Verification items for this drawing (mm, ordinates from the low corner). A direction names the side the tool comes from. Coordinates: 2 decimals unless noted, no trailing zeros. Loops run counter-clockwise (first coordinate to the right, second up) from the corner with the lowest first, then second, coordinate; pieces in that order, holes last. Notation, with made-up numbers: M 9,-23 L 66,-23 A17 cw 66,10 Z; hole C 76.5,51.25 d2. An arc over 180 degrees is marked long. Return JSON: item names as keys, results as strings.
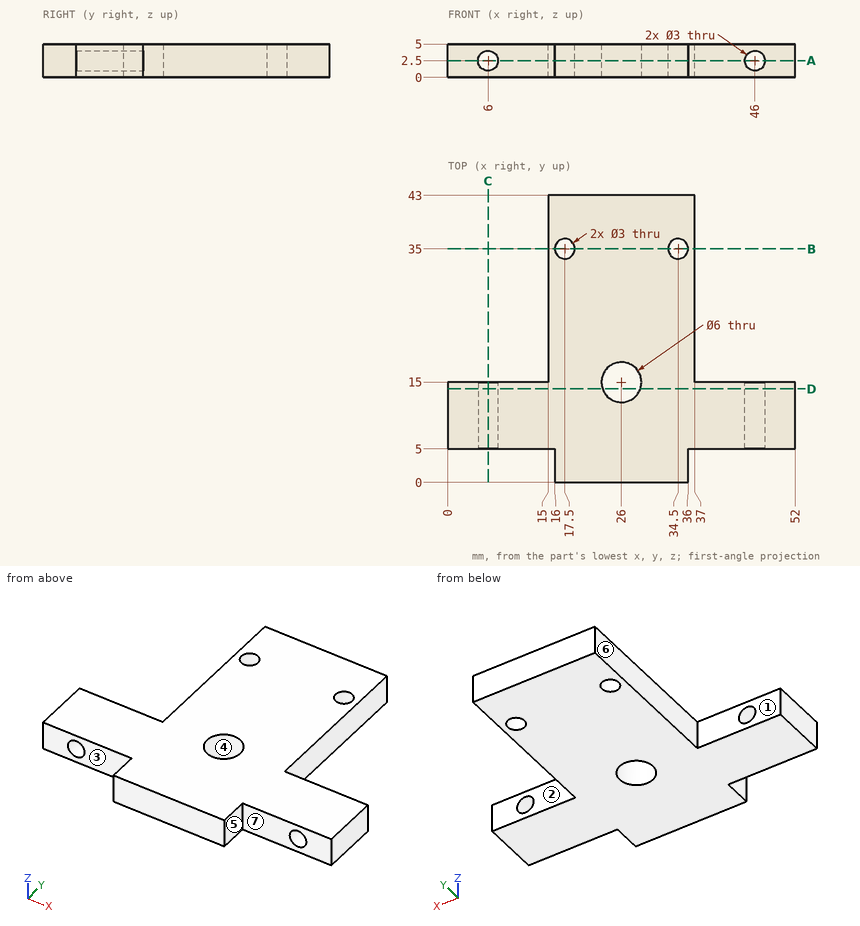
1) Draft check along X on the marked faces 4, 5, 6 and 7. Enter one of: +X half, -X half, draft (parallel to the pull), parting line (faces both ways), or undercut.
Answers:
{"face 4": "undercut", "face 5": "+X half", "face 6": "-X half", "face 7": "draft"}
2) Section check A-A on z = 2.5. Record the cut outline in (x, y).
Answers:
{"outline": "M 0,5 L 4.5,5 L 4.5,15 L 0,15 Z; M 7.5,5 L 16,5 L 16,0 L 36,0 L 36,5 L 44.5,5 L 44.5,15 L 37,15 L 37,43 L 15,43 L 15,15 L 7.5,15 Z; M 47.5,5 L 52,5 L 52,15 L 47.5,15 Z; hole C 17.5,35 d3; hole C 26,15 d6; hole C 34.5,35 d3"}
3) Set-up check for the marked faces 1, 2 and 3: record each of +Z, -Z, +X, -X, +Y, -Y from which the full face is reachable in a straight line by a thin tool's end or side.
Answers:
{"face 1": "+Z, -Z, -X, +Y", "face 2": "+Z, -Z, +X, +Y", "face 3": "+Z, -Z, -X, -Y"}
4) Section check D-D on y = 14. Record the cut outline in (x, z), then the cut area to 3 significant figures.
Answers:
{"outline": "M 0,0 L 23.17,0 L 23.17,5 L 0,5 Z; M 28.83,0 L 52,0 L 52,5 L 28.83,5 Z; hole C 6,2.5 d3; hole C 46,2.5 d3", "area": "218 mm²"}
5) Section check B-B on y = 35. Record the cut outline in (x, z).
Answers:
{"outline": "M 15,0 L 16,0 L 16,5 L 15,5 Z; M 19,0 L 33,0 L 33,5 L 19,5 Z; M 36,0 L 37,0 L 37,5 L 36,5 Z"}
6) Scan lines: line 1 along Y through (x, z) = (17.5, 1.8); line 2 along Y through (x, z) = (26, 2.65); line 3 along Y through (x, z) = (41.5, 3.9). Record each from-to range of solid material in increasing order. Write a range as [from, to].
Answers:
{"line 1": "[0, 33.5], [36.5, 43]", "line 2": "[0, 12], [18, 43]", "line 3": "[5, 15]"}
7) Go/stop test with flat-tipped pins: pin 1 Ø1 at (y, z) = (26.5, 4) entering from +X; pin 2 Ø2.5 at (x, z) = (46, 2.5) entering from +Y; pin 3 Ø1.5 at (y, z) = (28.5, 2.5) entering from -X; pin 4 Ø1.5 at (y, z) = (3, 3.5) entering from -X. Record where each tip stops, or that it passes through.
Answers:
{"pin 1": "x = 37", "pin 2": "through", "pin 3": "x = 15", "pin 4": "x = 16"}
8) Section check C-C on x = 6. Record the cut outline in (y, z).
Answers:
{"outline": "M 5,0 L 15,0 L 15,1 L 5,1 Z; M 5,4 L 15,4 L 15,5 L 5,5 Z"}
